Read the model definition and answer for the solid it produces. Units are mm, in the model's axes. A direction names the side the tool comes from. Give positions to 0.01 mm unless a question says otherwise; leave off trailing zeros. Loops run counter-clockwise (first coordinate to the right, second up) from the corner with the lowest first, then second, coordinate; pieces in that order, holes last. Notation, with made-up numbers: (50, -15.75) - (72, -15.75) arc R33 cw to (72, 16.25) - close; hole circle Ø1 at (-33.75, -20.5). An arc over 180 degrees is marked (long way). Write item = value, one per line.
```python
from build123d import *

# Parameters (mm, degrees)
SKETCH1_W           = 160
SKETCH1_H           = 40
BOSS_EXTRUDE1_DEPTH = 100
SKETCH2_W           = 7
SKETCH2_H           = 98.5
SKETCH2_W_2         = 15
CUT_EXTRUDE1_DEPTH  = 38
CUT_EXTRUDE2_DEPTH  = 2


with BuildPart() as part:
    # Sketch1 → Boss-Extrude1 (new body)
    with BuildSketch(Plane.XY):
        Rectangle(SKETCH1_W, SKETCH1_H)
    extrude(amount=BOSS_EXTRUDE1_DEPTH)

    # Sketch2 → Cut-Extrude1 (cut)
    with BuildSketch(Plane(origin=(0, 20, 0), x_dir=(1, 0, 0), z_dir=(0, 1, 0))):
        with Locations((-76.5, -50.75)):
            Rectangle(SKETCH2_W, SKETCH2_H)
        with Locations((72.5, -50.75)):
            Rectangle(SKETCH2_W_2, SKETCH2_H)
    extrude(amount=-CUT_EXTRUDE1_DEPTH, mode=Mode.SUBTRACT)

    # Sketch3 → Cut-Extrude2 (cut)
    with BuildSketch(Plane(origin=(0, -18, 0), x_dir=(1, 0, 0), z_dir=(0, 1, 0))):
        with BuildLine():
            Line((80, -4.5), (75, -4.5))
            ThreePointArc((75, -4.5), (73.5, -6), (75, -7.5))
            Line((75, -7.5), (80, -7.5))
            Line((80, -7.5), (80, -4.5))
        make_face()
        with BuildLine():
            Line((-80, -92.5), (-75, -92.5))
            ThreePointArc((-75, -92.5), (-73.5, -94), (-75, -95.5))
            Line((-75, -95.5), (-80, -95.5))
            Line((-80, -95.5), (-80, -92.5))
        make_face()
    extrude(amount=-CUT_EXTRUDE2_DEPTH, mode=Mode.SUBTRACT)


solid = part.part
```
1) Find the intervals of material crossed by probe 1 along X at (y, z) = (-15, 32); probe 2 along Y at (x, z) = (68, 96.5), in increasing order.
Output:
probe_1 = -73 to 65
probe_2 = -20 to -18
2) Each of these flat-tipped pins is pushed along its axis until it touches: P1, Ø3.5, axis at x = -77.5, y = -5, coming from the +Z side; P2, Ø5.5, axis at x = -78, z = 49, coming from the +Y side; P3, Ø5, axis at y = 7, z = 54, coming from the -X side. Where does it stop, or does it pass through?
Output:
P1 = 1.5
P2 = -18
P3 = -73
3) A tool of negligible diameter and unlimited length cuts with its end or side. For faces 1 (the face through (-80, -19, 25)), 2 (the face through (72, 1, 1.5)), 3 (the face through (-77, -18, 50)), from which of +Z, -Z, +X, -X, +Y, -Y can it reach the whole face along a straight path? Write none if from no direction.
Output:
face_1 = +Z, -Z, -X, +Y, -Y
face_2 = +Z, +X, +Y
face_3 = +Z, -X, +Y
4) A cutting plane is placed at A-A on y = 17. Determine the outline of the cut face in (x, z).
Output:
outline = (-80, 0) - (80, 0) - (80, 1.5) - (65, 1.5) - (65, 100) - (-73, 100) - (-73, 1.5) - (-80, 1.5) - close
5) A cutting plane is placed at B-B on z = 18. Determine the outline of the cut face in (x, y), then the cut area to 3 significant figures.
Output:
outline = (-80, -20) - (80, -20) - (80, -18) - (65, -18) - (65, 20) - (-73, 20) - (-73, -18) - (-80, -18) - close
area = 5,560 mm²
